```python
from build123d import *

# Parameters (mm, degrees)
F0_W     = 110
F0_H     = 40
F1_DEPTH = 25
F2_R     = 12.5
F3_DEPTH = 24.5
F4_R     = 5
F5_DEPTH = 25
F6_DEPTH = 25


with BuildPart() as f1:
    # F0 (on Right) → F1 (new body)
    with BuildSketch(Plane.YZ):
        with Locations((0, -4.401192)):
            Rectangle(F0_W, F0_H)
    extrude(amount=F1_DEPTH)

    # F2 (on face) → F3 (join)
    with BuildSketch(Plane(origin=(0, 0, 0), x_dir=(0, -1, 0), z_dir=(-1, 0, 0))):
        with Locations((-5, -4.401192)):
            Circle(F2_R)
    extrude(amount=F3_DEPTH)

    # F4 (on face) → F5 (cut)
    with BuildSketch(Plane.XZ.offset(55)):
        with Locations((12.5, 5.598808)):
            Circle(F4_R)
    extrude(amount=-F5_DEPTH, mode=Mode.SUBTRACT)

    # F4 (on face) → F6 (cut)
    with BuildSketch(Plane.XZ.offset(55)):
        with Locations((12.5, 5.598808)):
            Circle(F4_R)
        with Locations((12.5, -14.401192)):
            Circle(F4_R)
    extrude(amount=-F6_DEPTH, mode=Mode.SUBTRACT)


solid = f1.part
```
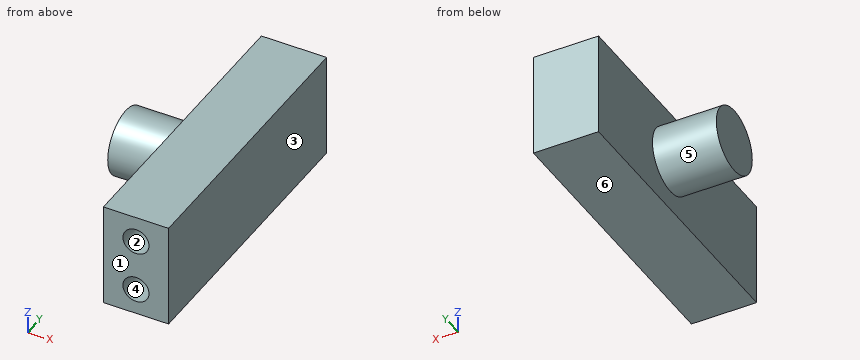
Could you check a few things on this model? Use its own coordinates, in mm. Face numbers are marked on the shaded views. A direction names the side the tool comes from. Round coordinates to 2 decimals unless told otherwise and drop trailing zeros. Loops run counter-clockwise (first coordinate to the right, second up) from the corner with the lowest first, then second, coordinate; pieces in that order, holes last.
Q1. Thinking about a two-plate mould opening in Z: for the marked faces 3, 4, 5 and 6, which applies, pulls with the +Z half, pulls with the -Z half, needs draft (parallel to the pull), parting line crosses it, or undercut?
Q2. Please list where these lines run through material, in increasing order: L1, parallel to Z at x = 12.5, y = -42.25; L2, parallel to X at y = -50, z = -8; L3, parallel to Y at x = 11, z = 8.
Q3. I want a section at B-B (x = 12.5). Write out the boundary of the cut face in (y, z), and give its area (3 significant figures).
Q4. I want a section at D-D (x = -3.5). Write out the boundary of the cut face in (y, z), and give its area (3 significant figures).
Q5. On a 3-axis mill with a long thin cutter (end or side, diameter ignored), from which of +Z, -Z, +X, -X, +Y, -Y can I reach the whole of each face in a straight line? I mean the marked faces 1 and 2. Say none if no direction works.
Q6. I want a section at A-A (y = 5). Write out the boundary of the cut face in (x, z), and give its area (3 significant figures).
Q7. For P1, Ø12, axis at y = -31, z = 0, coming from the -X side; P2, Ø3, axis at x = 13.5, z = 6, coming from the -Y side; P3, Ø3, axis at x = -11.5, z = 4, coming from the -Y side, each with a flat end and sliding along its axis, tell me the tip position at first contact or that it passes through.
Q8. I want a section at C-C (y = -16). Write out the boundary of the cut face in (x, z).
Answer below:
1. face 3: needs draft
1. face 4: undercut
1. face 5: parting line crosses it
1. face 6: pulls with the -Z half
2. L1: z = -24.4 to -19.4, -9.4 to 0.6, 10.6 to 15.6
2. L2: x = 0 to 25
2. L3: y = -30 to 55
3. outline: (-55, -24.4) - (55, -24.4) - (55, 15.6) - (-55, 15.6) - (-55, 10.6) - (-30, 10.6) - (-30, 0.6) - (-55, 0.6) - (-55, -9.4) - (-30, -9.4) - (-30, -19.4) - (-55, -19.4) - close
3. area: 3,900 mm2
4. outline: circle Ø25 at (5, -4.4)
4. area: 491 mm2
5. face 1: +Z, -Z, +X, -X, -Y
5. face 2: -Y
6. outline: (-24.5, -16.9) - (0, -16.9) - (0, -24.4) - (25, -24.4) - (25, 15.6) - (0, 15.6) - (0, 8.1) - (-24.5, 8.1) - close
6. area: 1,610 mm2
7. P1: stops at x = 0
7. P2: stops at y = -30
7. P3: stops at y = -5.42
8. outline: (0, -24.4) - (25, -24.4) - (25, 15.6) - (0, 15.6) - close
